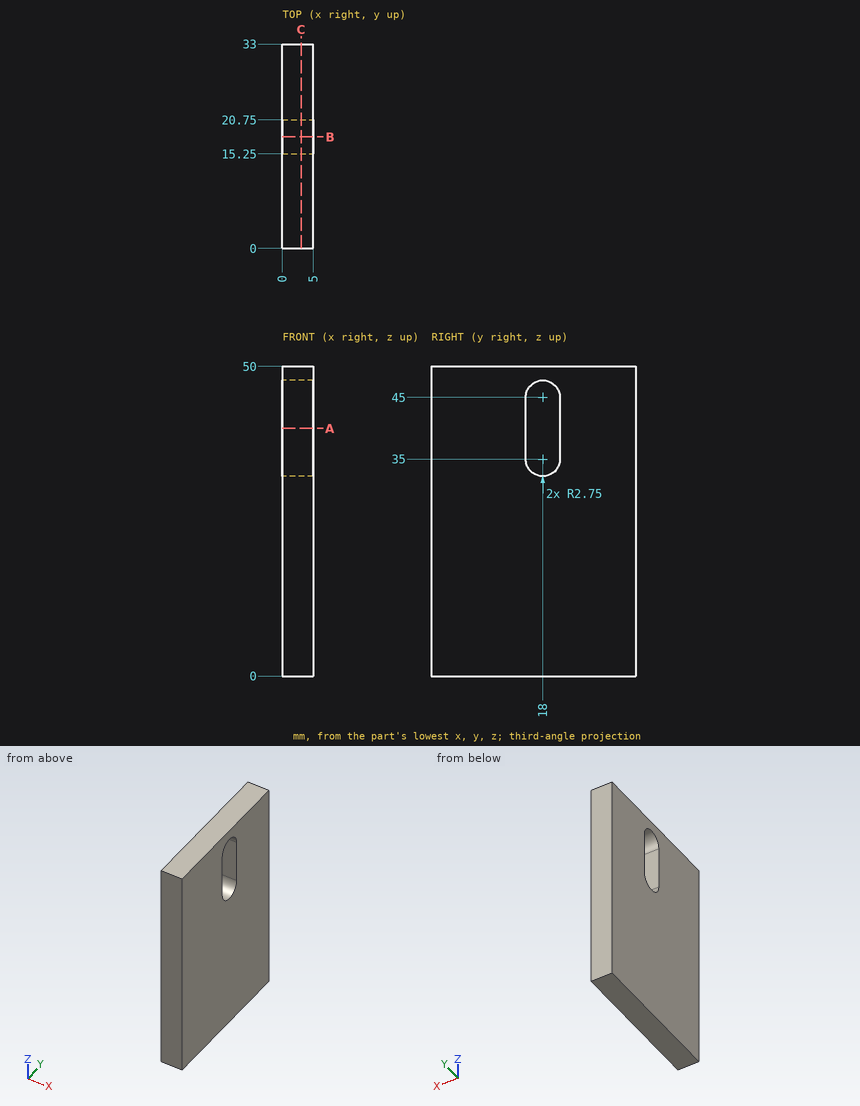
Verification items for this drawing (mm, ordinates from the low corner). Round coordinates to 2 decimals unless told otherwise and drop trailing zeros. Loops run counter-clockwise (first coordinate to the right, second up) from the corner with the lowest first, then second, coordinate; pieces in that order, holes last. Notation, with made-up numbers: (-13.5, 37) - (21.5, 37) arc R35 cw to (21.5, 75) - close; hole circle Ø4 at (69, 5). An arc over 180 degrees is marked (long way). Write item = value, one per line.
Q1. Sectioned sample at C-C on x = 3.05. Record the boundary of the cut face in (y, z), plus the area to 3 significant figures.
Here are the results:
outline = (0, 0) - (33, 0) - (33, 50) - (0, 50) - close; hole (15.25, 35) arc R2.75 ccw to (20.75, 35) - (20.75, 45) arc R2.75 ccw to (15.25, 45) - close
area = 1,570 mm^2
Q2. Sectioned sample at A-A on z = 40. Record the boundary of the cut face in (x, y).
Here are the results:
outline = (0, 0) - (5, 0) - (5, 15.25) - (0, 15.25) - close; (0, 20.75) - (5, 20.75) - (5, 33) - (0, 33) - close
Q3. Sectioned sample at B-B on y = 18. Record the boundary of the cut face in (x, z).
Here are the results:
outline = (0, 0) - (5, 0) - (5, 32.25) - (0, 32.25) - close; (0, 47.75) - (5, 47.75) - (5, 50) - (0, 50) - close
Q4. Material ranges on L1, parallel to Y at x = 0.8, z = 36; L2, parallel to Z at x = 0.8, y = 18; L3, parallel to Y at x = 3.15, z = 45.5, recorded low to high.
Here are the results:
L1 = 0 to 15.25, 20.75 to 33
L2 = 0 to 32.25, 47.75 to 50
L3 = 0 to 15.3, 20.7 to 33
